```python
from build123d import *

# Parameters (mm, degrees)
SKETCH_1_R      = 5
EXTRUDE_1_DEPTH = 10
SKETCH_2_W      = 20
SKETCH_2_H      = 20
EXTRUDE_2_DEPTH = 5


with BuildPart() as part:
    # 草图1 → 凸台-拉伸1 (new, symmetric)
    with BuildSketch(Plane.XY):
        Circle(SKETCH_1_R)
    extrude(amount=EXTRUDE_1_DEPTH, both=True)

    # 草图2 → 凸台-拉伸2 (add)
    with BuildSketch(Plane(origin=(0, 0, -10), x_dir=(-1, 0, 0), z_dir=(0, 0, -1))):
        Rectangle(SKETCH_2_W, SKETCH_2_H)
    extrude(amount=EXTRUDE_2_DEPTH)


solid = part.part
```
Part model, mm, in its own coordinate system. A direction names the side the tool comes from. Coordinates: 2 decimals unless noted, no trailing zeros. Order: outer loops, then holes, each group sorted by start corner. A loop starts at its lowest first (then second) coordinate and runs counter-clockwise, first axis right, second up. Notation, with made-up numbers: (80.5, 24) - (98.5, 24) arc R20 cw to (98.5, 34) - close; hole circle Ø2 at (76, 1). An arc over 180 degrees is marked (long way). Return JSON: item names as keys, results as strings. Group by question number.
Item 1: Cut at C-C (z = -8.75). List the corners of the cut face in (x, y).
Item 2: Drill centre lines: probe 1 along Z at (x, y) = (-3.25, -4.5); probe 2 along X at (y, z) = (3.75, 6); probe 3 along X at (y, z) = (2.5, -4). Where is each one in solid material? Low to high. Write a range as from..to.
Item 3: Which spindle directions (+Z, -Z, +X, -X, +Y, -Y) get a long thin tool onto all of the face, cutting with end or side? Do faces 1 (the face through (2, 5, -10)), 2 (the face through (0, 10, -12)). Say none if no direction does.
Item 4: Pin check, flat tips, straight feed: pin 1 (12 mm diameter, centred on x = -0.5, z = 6, fed in from +Y); pin 2 (1 mm diameter, centred on x = 1.5, z = 1.5, fed in from -Y); pin 3 (6 mm diameter, centred on y = 6.5, z = -6, fed in from +X). Stop position of each tip, or through.
Item 5: Cut at D-D (x = 7.75). List the corners of the cut face in (y, z).
Item 6: Cut at A-A (y = 0). List the corners of the cut face in (x, z).
Check values:
{
 "1": {"outline": "circle Ø10 at (0, 0)"},
 "2": {"probe 1": "z = -15..-10", "probe 2": "x = -3.31..3.31", "probe 3": "x = -4.33..4.33"},
 "3": {"face 1": "+Z", "face 2": "+Z, -Z, +X, -X, +Y"},
 "4": {"pin 1": "stops at y = 5", "pin 2": "stops at y = -4.9", "pin 3": "stops at x = 3.57"},
 "5": {"outline": "(-10, -15) - (10, -15) - (10, -10) - (-10, -10) - close"},
 "6": {"outline": "(-10, -15) - (10, -15) - (10, -10) - (5, -10) - (5, 10) - (-5, 10) - (-5, -10) - (-10, -10) - close"}
}
